Check sheet for the modelled part. Datum: model origin and axes. Units: mm. Face numbers are marked on the shaded views. Round coordinates to 2 decimals unless told otherwise and drop trailing zeros.
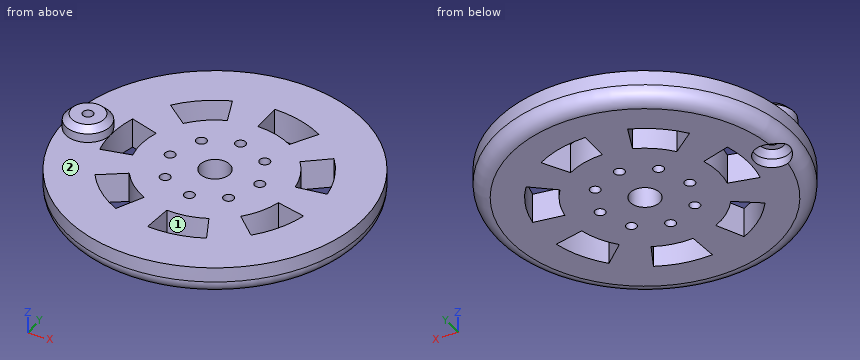
```python
from build123d import *

# Parameters (mm, degrees)
SKETCH1_R           = 50
BOSS_EXTRUDE1_DEPTH = 10
SKETCH2_R           = 5
CUT_EXTRUDE1_DEPTH  = 72.414284285
FILLET1_R           = 5
SKETCH3_R           = 1.75
CUT_EXTRUDE2_DEPTH  = 72.414284425
SKETCH5_R           = 7.5
BOSS_EXTRUDE2_DEPTH = 5
SKETCH6_R           = 1.75
CUT_EXTRUDE3_DEPTH  = 73.284161612
SKETCH7_R           = 5.939963611
CUT_EXTRUDE4_DEPTH  = 5
CHAMFER1_SIZE       = 2
CHAMFER2_SIZE       = 2
CUT_EXTRUDE5_DEPTH  = 72.414284439
CIRPATTERN1_COUNT   = 7


with BuildPart() as part:
    # Sketch1 → Boss-Extrude1 (new body)
    with BuildSketch(Plane.XY):
        Circle(SKETCH1_R)
    extrude(amount=BOSS_EXTRUDE1_DEPTH)

    # Sketch2 → Cut-Extrude1 (cut, through all)
    with BuildSketch(Plane.XY.offset(10)):
        Circle(SKETCH2_R)
    extrude(amount=-CUT_EXTRUDE1_DEPTH, mode=Mode.SUBTRACT)

    # Fillet1
    fillet1_edges = [part.edges().sort_by_distance(p)[0] for p in [
        (-50, 0, 0),
    ]]
    fillet(fillet1_edges, radius=FILLET1_R)

    # Sketch3 → Cut-Extrude2 (cut, through all)
    with BuildSketch(Plane(origin=(0, 0, 0), x_dir=(-1, 0, 0), z_dir=(0, 0, -1))):
        with Locations((0, 15)):
            Circle(SKETCH3_R)
        with Locations((10.606601718, 10.606601718)):
            Circle(SKETCH3_R)
        with Locations((15, 0)):
            Circle(SKETCH3_R)
        with Locations((10.606601718, -10.606601718)):
            Circle(SKETCH3_R)
        with Locations((0, -15)):
            Circle(SKETCH3_R)
        with Locations((-10.606601718, -10.606601718)):
            Circle(SKETCH3_R)
        with Locations((-15, 0)):
            Circle(SKETCH3_R)
        with Locations((-10.606601718, 10.606601718)):
            Circle(SKETCH3_R)
    extrude(amount=-CUT_EXTRUDE2_DEPTH, mode=Mode.SUBTRACT)

    # Sketch5 → Boss-Extrude2 (add)
    with BuildSketch(Plane.XY.offset(10)):
        with Locations(Location((-42.5, 0, 0), (0, 0, 179.999679023))):
            Circle(SKETCH5_R)
    extrude(amount=BOSS_EXTRUDE2_DEPTH)

    # Sketch6 → Cut-Extrude3 (cut, through all)
    with BuildSketch(Plane.XY.offset(15)):
        with Locations((-42.5, 0)):
            Circle(SKETCH6_R)
    extrude(amount=-CUT_EXTRUDE3_DEPTH, mode=Mode.SUBTRACT)

    # Sketch7 → Cut-Extrude4 (cut)
    with BuildSketch(Plane(origin=(0, 0, 0), x_dir=(-1, 0, 0), z_dir=(0, 0, -1))):
        with Locations((42.5, 0)):
            Circle(SKETCH7_R)
    extrude(amount=-CUT_EXTRUDE4_DEPTH, mode=Mode.SUBTRACT)

    # Chamfer1
    chamfer1_edges = [part.edges().sort_by_distance(p)[0] for p in [
        (-36.560036389, 0, 5),
    ]]
    chamfer(chamfer1_edges, length=CHAMFER1_SIZE)

    # Chamfer2
    chamfer2_edges = [part.edges().sort_by_distance(p)[0] for p in [
        (-35, -4.2016e-05, 15),
    ]]
    chamfer(chamfer2_edges, length=CHAMFER2_SIZE)

    # Sketch8 → Cut-Extrude5 (cut, through all)
    with BuildSketch(Plane.XY.offset(10)):
        with BuildLine():
            Line((0, 35), (0, 25))
            ThreePointArc((0, 25), (6.470476128, 24.148145657), (12.5, 21.650635095))
            Line((12.5, 21.650635095), (17.5, 30.310889132))
            ThreePointArc((17.5, 30.310889132), (9.058666579, 33.80740392), (0, 35))
        make_face()
    cut_extrude5 = extrude(amount=-CUT_EXTRUDE5_DEPTH, mode=Mode.SUBTRACT)

    # CirPattern1: Cut-Extrude5 ×7 about axis
    cirpattern1_axis = Axis((0, 0, 0), (0, 0, 1))
    for i in range(1, CIRPATTERN1_COUNT):
        add(cut_extrude5.rotate(cirpattern1_axis, i * 360 / CIRPATTERN1_COUNT), mode=Mode.SUBTRACT)


solid = part.part
```
Item 1: Sectioned sample at A-A (z = 7.75). State how many separate pieces and enclosed holes the cut face has, and give its area (3 significant figures).
Answer:
separate pieces: 1
enclosed holes: 17
area: 6,590 mm2
Item 2: Go/stop test with flat-tipped pins: P1, Ø4, axis at x = -10.61, y = -10.61, coming from the +Z side; P2, Ø3, axis at y = -14, z = 9, coming from the +X side; P3, Ø3, axis at y = 29, z = 3, coming from the +X side. Record where each tip stops, or that it passes through.
Answer:
P1: stops at z = 10
P2: stops at x = 48.41
P3: stops at x = 41.44
Item 3: Scan lines: line 1 along X through (y, z) = (0.5, 8.5) (1 decimal); line 2 along Y through (x, z) = (15, 8); line 3 along Z through (x, y) = (2.5, 7.5). Record each from-to range of solid material in increasing order.
Answer:
line 1: x = -50 to -44.2, -40.8 to -35, -25 to -16.7, -13.3 to -5, 5 to 13.3, 16.7 to 50
line 2: y = -47.7 to -31.62, -31.15 to -1.75, 1.75 to 25.98, 31.62 to 47.7
line 3: z = 0 to 10
Item 4: Release check for a two-part mould opening along Y. For the marked faces 1 and 2 record: released by +Y, released by -Y, zero draft, split by the parting line, or undercut.
Answer:
face 1: undercut
face 2: zero draft
